Check sheet for the modelled part. Datum: model origin and axes. Units: mm. Face numbers are marked on the shaded views. A direction names the side the tool comes from. Round coordinates to 2 decimals unless told otherwise and drop trailing zeros. Order: outer loops, then holes, each group sorted by start corner. A loop starts at its lowest first (then second) coordinate and runs counter-clockwise, first axis right, second up. Notation, with made-up numbers: (24.5, -9.75) -> (45.5, -9.75) arc R19 ccw to (45.5, 22.25) -> close; hole circle Ø2 at (8, 20.25). An arc over 180 degrees is marked (long way). Answer in a Markdown table with one row per item. Add a question column.
1. Access from +Z, -Z, +X, -X, +Y, -Y to the whole of each face (thin tool, end or side, straight path). Record for the marked faces 5, 6, 7 and 8.
2. Draft check along Y on the marked faces 1, 2, 3 and 4. Enter one of: +Y half, -Y half, draft (parallel to the pull), parting line (faces both ways), or undercut.
3. Sectioned sample at A-A, the plane y = 0. Record the boundary of the cut face in (x, z).
4. Material ranges on L1, parallel to Y at x = 6.75, z = 3.25; L2, parallel to X at y = -6.5, z = 3; L3, parallel to Y at x = -7.5, z = 2, recorded low to high. Write a range as from..to.
5. Sectioned sample at B-B, the plane x = 0. Record the boundary of the cut face in (y, z).
6. Depth check by flat-ended pin: P1, Ø3, axis at x = 1, y = 1.5, coming from the +Z side; P2, Ø5, axis at y = -6, z = 6, coming from the -X side; P3, Ø1, axis at y = -3.5, z = 6.5, coming from the -X side. Enter the tip coordinate at first touch or a pass-through.
7. Sectioned sample at C-C, the plane y = -5. Record the boundary of the cut face in (x, z), then the cut area to 3 significant figures.
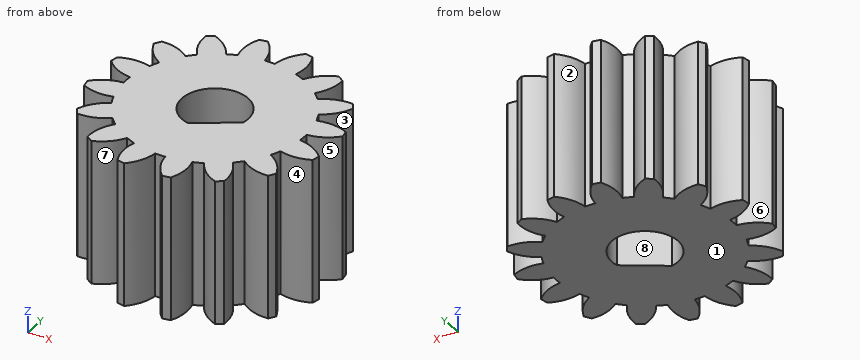
```python
from build123d import *

# Parameters (mm, degrees)
BOSS_EXTRUDE1_DEPTH = 10


with BuildPart() as part:
    # Model → Boss-Extrude1 (new body)
    with BuildSketch(Plane.XY):
        with BuildLine():
            ThreePointArc((-8.115592249, 1.337081693), (-7.243390826, 0.66756543), (-6.188733379, 0.356623286))
            ThreePointArc((-6.188733379, 0.356623286), (-6.199, 0), (-6.188733379, -0.356623286))
            ThreePointArc((-6.188733379, -0.356623286), (-7.243390826, -0.66756543), (-8.115592249, -1.337081693))
            ThreePointArc((-8.115592249, -1.337081693), (-8.066958931, -1.604617899), (-8.009508584, -1.870400288))
            ThreePointArc((-8.009508584, -1.870400288), (-6.94748676, -2.155175626), (-5.854117924, -2.038848777))
            ThreePointArc((-5.854117924, -2.038848777), (-5.727129222, -2.372254597), (-5.581170278, -2.697802686))
            ThreePointArc((-5.581170278, -2.697802686), (-6.4365543, -3.388675701), (-6.986150561, -4.341005107))
            ThreePointArc((-6.986150561, -4.341005107), (-6.838837561, -4.569565167), (-6.684049844, -4.793130781))
            ThreePointArc((-6.684049844, -4.793130781), (-5.593890814, -4.649810729), (-4.628266083, -4.123924595))
            ThreePointArc((-4.628266083, -4.123924595), (-4.383354937, -4.383354937), (-4.123924596, -4.628266083))
            ThreePointArc((-4.123924596, -4.628266083), (-4.649810729, -5.593890814), (-4.793130781, -6.684049844))
            ThreePointArc((-4.793130781, -6.684049844), (-4.569565167, -6.838837561), (-4.341005107, -6.986150561))
            ThreePointArc((-4.341005107, -6.986150561), (-3.388675701, -6.4365543), (-2.697802686, -5.581170278))
            ThreePointArc((-2.697802686, -5.581170278), (-2.372254597, -5.727129222), (-2.038848777, -5.854117924))
            ThreePointArc((-2.038848777, -5.854117924), (-2.155175626, -6.94748676), (-1.870400288, -8.009508584))
            ThreePointArc((-1.870400288, -8.009508584), (-1.604617899, -8.066958931), (-1.337081693, -8.115592249))
            ThreePointArc((-1.337081693, -8.115592249), (-0.66756543, -7.243390826), (-0.356623286, -6.188733379))
            ThreePointArc((-0.356623286, -6.188733379), (0, -6.199), (0.356623286, -6.188733379))
            ThreePointArc((0.356623286, -6.188733379), (0.66756543, -7.243390826), (1.337081693, -8.115592249))
            ThreePointArc((1.337081693, -8.115592249), (1.604617899, -8.066958931), (1.870400288, -8.009508584))
            ThreePointArc((1.870400288, -8.009508584), (2.155175626, -6.94748676), (2.038848777, -5.854117924))
            ThreePointArc((2.038848777, -5.854117924), (2.372254597, -5.727129222), (2.697802686, -5.581170278))
            ThreePointArc((2.697802686, -5.581170278), (3.388675701, -6.4365543), (4.341005107, -6.986150561))
            ThreePointArc((4.341005107, -6.986150561), (4.569565167, -6.838837561), (4.793130781, -6.684049844))
            ThreePointArc((4.793130781, -6.684049844), (4.649810729, -5.593890814), (4.123924595, -4.628266083))
            ThreePointArc((4.123924595, -4.628266083), (4.383354937, -4.383354937), (4.628266083, -4.123924595))
            ThreePointArc((4.628266083, -4.123924595), (5.593890814, -4.649810729), (6.684049844, -4.79313078))
            ThreePointArc((6.684049844, -4.79313078), (6.838837561, -4.569565167), (6.986150561, -4.341005107))
            ThreePointArc((6.986150561, -4.341005107), (6.4365543, -3.388675701), (5.581170278, -2.697802686))
            ThreePointArc((5.581170278, -2.697802686), (5.727129222, -2.372254597), (5.854117924, -2.038848777))
            ThreePointArc((5.854117924, -2.038848777), (6.94748676, -2.155175626), (8.009508584, -1.870400288))
            ThreePointArc((8.009508584, -1.870400288), (8.066958931, -1.604617899), (8.115592249, -1.337081693))
            ThreePointArc((8.115592249, -1.337081693), (7.243390826, -0.66756543), (6.188733379, -0.356623286))
            ThreePointArc((6.188733379, -0.356623286), (6.199, 0), (6.188733379, 0.356623286))
            ThreePointArc((6.188733379, 0.356623286), (7.243390826, 0.66756543), (8.115592249, 1.337081693))
            ThreePointArc((8.115592249, 1.337081693), (8.066958931, 1.604617899), (8.009508584, 1.870400288))
            ThreePointArc((8.009508584, 1.870400288), (6.94748676, 2.155175626), (5.854117924, 2.038848777))
            ThreePointArc((5.854117924, 2.038848777), (5.727129222, 2.372254597), (5.581170278, 2.697802686))
            ThreePointArc((5.581170278, 2.697802686), (6.4365543, 3.388675701), (6.986150561, 4.341005107))
            ThreePointArc((6.986150561, 4.341005107), (6.838837561, 4.569565167), (6.684049844, 4.793130781))
            ThreePointArc((6.684049844, 4.793130781), (5.593890814, 4.649810729), (4.628266083, 4.123924595))
            ThreePointArc((4.628266083, 4.123924595), (4.383354937, 4.383354937), (4.123924595, 4.628266083))
            ThreePointArc((4.123924595, 4.628266083), (4.649810729, 5.593890814), (4.79313078, 6.684049844))
            ThreePointArc((4.79313078, 6.684049844), (4.569565167, 6.838837561), (4.341005107, 6.986150561))
            ThreePointArc((4.341005107, 6.986150561), (3.388675701, 6.4365543), (2.697802686, 5.581170278))
            ThreePointArc((2.697802686, 5.581170278), (2.372254597, 5.727129222), (2.038848777, 5.854117924))
            ThreePointArc((2.038848777, 5.854117924), (2.155175626, 6.94748676), (1.870400288, 8.009508584))
            ThreePointArc((1.870400288, 8.009508584), (1.604617899, 8.066958931), (1.337081693, 8.115592249))
            ThreePointArc((1.337081693, 8.115592249), (0.66756543, 7.243390826), (0.356623286, 6.188733379))
            ThreePointArc((0.356623286, 6.188733379), (0, 6.199), (-0.356623286, 6.188733379))
            ThreePointArc((-0.356623286, 6.188733379), (-0.66756543, 7.243390826), (-1.337081693, 8.115592249))
            ThreePointArc((-1.337081693, 8.115592249), (-1.604617899, 8.066958931), (-1.870400288, 8.009508584))
            ThreePointArc((-1.870400288, 8.009508584), (-2.155175626, 6.94748676), (-2.038848777, 5.854117924))
            ThreePointArc((-2.038848777, 5.854117924), (-2.372254597, 5.727129222), (-2.697802686, 5.581170278))
            ThreePointArc((-2.697802686, 5.581170278), (-3.388675701, 6.4365543), (-4.341005107, 6.986150561))
            ThreePointArc((-4.341005107, 6.986150561), (-4.569565167, 6.838837561), (-4.793130781, 6.684049844))
            ThreePointArc((-4.793130781, 6.684049844), (-4.649810729, 5.593890814), (-4.123924595, 4.628266083))
            ThreePointArc((-4.123924595, 4.628266083), (-4.383354937, 4.383354937), (-4.628266083, 4.123924595))
            ThreePointArc((-4.628266083, 4.123924595), (-5.593890814, 4.649810729), (-6.684049844, 4.79313078))
            ThreePointArc((-6.684049844, 4.79313078), (-6.838837561, 4.569565167), (-6.986150561, 4.341005107))
            ThreePointArc((-6.986150561, 4.341005107), (-6.4365543, 3.388675701), (-5.581170278, 2.697802686))
            ThreePointArc((-5.581170278, 2.697802686), (-5.727129222, 2.372254597), (-5.854117924, 2.038848777))
            ThreePointArc((-5.854117924, 2.038848777), (-6.94748676, 2.155175626), (-8.009508584, 1.870400288))
            ThreePointArc((-8.009508584, 1.870400288), (-8.066958931, 1.604617899), (-8.115592249, 1.337081693))
        make_face()
        with BuildLine():
            Line((-0.506237517, -2.243596126), (2.256391081, -0.445756983))
            ThreePointArc((2.256391081, -0.445756983), (-1.254518143, 1.927740706), (-0.506237517, -2.243596126))
        make_face(mode=Mode.SUBTRACT)
    extrude(amount=BOSS_EXTRUDE1_DEPTH)


solid = part.part
```
Answer key:
| question | item | result |
|---|---|---|
| 1 | face 5 | +Z, -Z, +X |
| 1 | face 6 | +Z, -Z, -X |
| 1 | face 7 | +Z, -Z, -Y |
| 1 | face 8 | +Z, -Z |
| 2 | face 1 | draft |
| 2 | face 2 | +Y half |
| 2 | face 3 | undercut |
| 2 | face 4 | undercut |
| 3 | outline | (-6.2, 0) -> (-2.3, 0) -> (-2.3, 10) -> (-6.2, 10) -> close; (2.3, 0) -> (6.2, 0) -> (6.2, 10) -> (2.3, 10) -> close |
| 4 | L1 | y = -4.7..-3.83, -2.16..-0.47, 0.47..2.16, 3.83..4.7 |
| 4 | L2 | x = -4.8..-3.47, -2.16..-0.41, 0.41..2.16, 3.47..4.8 |
| 4 | L3 | y = -2.06..-0.81, 0.81..2.06 |
| 5 | outline | (-6.2, 0) -> (-1.91, 0) -> (-1.91, 10) -> (-6.2, 10) -> close; (2.3, 0) -> (6.2, 0) -> (6.2, 10) -> (2.3, 10) -> close |
| 6 | P1 | stops at z = 10 |
| 6 | P2 | stops at x = -6.99 |
| 6 | P3 | stops at x = -6.84 |
| 7 | outline | (-4.38, 0) -> (4.38, 0) -> (4.38, 10) -> (-4.38, 10) -> close |
| 7 | area | 87.6 mm² |
